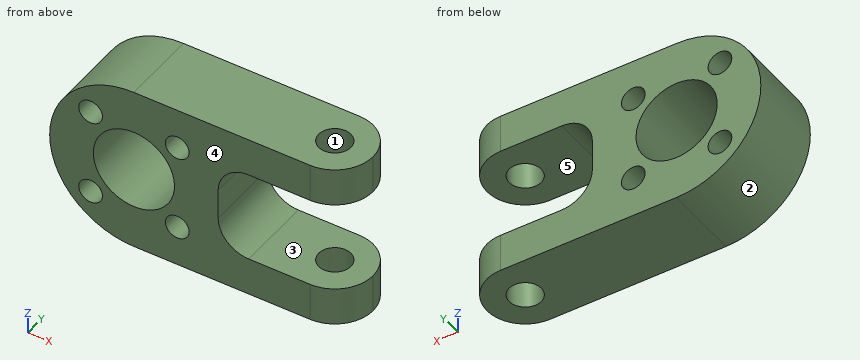
```python
from build123d import *

# Parameters (mm, degrees)
SKETCH2_R           = 5.3
SKETCH2_R_2         = 1.55
BOSS_EXTRUDE2_DEPTH = 10
SKETCH7_R           = 2.1
CUT_EXTRUDE2_DEPTH  = 46.880278988
FILLET1_R           = 4


with BuildPart() as part:
    # Sketch2 → Boss-Extrude2 (new body)
    with BuildSketch(Plane(origin=(0, 0, 0), x_dir=(1, 0, 0), z_dir=(0, 1, 0))):
        with BuildLine():
            Line((-28, -11), (0, -11))
            Line((0, -11), (0, -6))
            Line((0, -6), (-17, -6))
            Line((-17, -6), (-17, 6))
            Line((-17, 6), (0, 6))
            Line((0, 6), (0, 11))
            Line((0, 11), (-28, 11))
            ThreePointArc((-28, 11), (-39, 0), (-28, -11))
        make_face()
        with Locations(Location((-28, 0, 0), (0, 0, 270))):
            Circle(SKETCH2_R, mode=Mode.SUBTRACT)
        with Locations(Location((-33.656854249, 5.656854249, 0), (0, 0, 270))):
            Circle(SKETCH2_R_2, mode=Mode.SUBTRACT)
        with Locations(Location((-33.656854249, -5.656854249, 0), (0, 0, 270))):
            Circle(SKETCH2_R_2, mode=Mode.SUBTRACT)
        with Locations(Location((-22.343145751, 5.656854249, 0), (0, 0, 270))):
            Circle(SKETCH2_R_2, mode=Mode.SUBTRACT)
        with Locations(Location((-22.343145751, -5.656854249, 0), (0, 0, 270))):
            Circle(SKETCH2_R_2, mode=Mode.SUBTRACT)
    extrude(amount=BOSS_EXTRUDE2_DEPTH)

    # Sketch7 → Cut-Extrude2 (cut, through all)
    with BuildSketch(Plane.XY.offset(11)):
        with BuildLine():
            Line((0, 10), (-5, 10))
            ThreePointArc((-5, 10), (-1.464466094, 8.535533906), (0, 5))
            Line((0, 5), (0, 10))
        make_face()
        with BuildLine():
            Line((0, 0), (0, 5))
            ThreePointArc((0, 5), (-1.464466094, 1.464466094), (-5, 0))
            Line((-5, 0), (0, 0))
        make_face()
        with Locations((-5, 5)):
            Circle(SKETCH7_R)
    extrude(amount=-CUT_EXTRUDE2_DEPTH, mode=Mode.SUBTRACT)

    # Fillet1
    fillet1_edges = [part.edges().sort_by_distance(p)[0] for p in [
        (-17, 5, 6),
        (-17, 5, -6),
    ]]
    fillet(fillet1_edges, radius=FILLET1_R)


solid = part.part
```
Geometry check sheet. Reference: the model listing, model coordinates, mm. Face numbers are marked on the shaded views. A direction names the side the tool comes from. Give positions to 0.01 mm unless a question says otherwise; leave off trailing zeros. Order: outer loops, then holes, each group sorted by start corner. A loop starts at its lowest first (then second) coordinate and runs counter-clockwise, first axis right, second up. Notation, with made-up numbers: (54.25, -12.5) - (100.25, -12.5) arc R31 ccw to (100.25, 21.5) - close; hole circle Ø11 at (-26.75, 88). An arc over 180 degrees is marked (long way). Answer in a Markdown table with one row per item. Add a question column.
Q1. Cross-section at C-C, the plane z = -1.5. Enter the section's corners in (x, y), then the cut area to 3 significant figures.
Q2. Material ranges on probe 1 along Z at (x, y) = (-9, 5); probe 2 along Y at (x, z) = (-5, 7.75); probe 3 along Z at (x, y) = (-35, 8), recorded low to high. Write a range as from..to.
Q3. Tool access check on the marked faces 4 and 5. Record the directions out of +Z, -Z, +X, -X, +Y, -Y that give a thin tool (end or side, any length) a straight path to the whole face; none if there is none.
Q4. Cross-section at A-A, the plane y = 9. Enter the section's corners in (x, z).
Q5. Cross-section at D-D, the plane y = 1.75. Enter the section's corners in (x, z).
Q6. Gauge pin test, flat ends, axial feed: pin 1 (8 mm diameter, centred on x = -17, z = -8.5, fed in from -Y); pin 2 (1.9 mm diameter, centred on x = -22.34, z = -5.66, fed in from +Y); pin 3 (4.5 mm diameter, centred on y = 5.5, z = -0.5, fed in from +X). Record the tip position at first contact, or that the pin passes through.
Q7. Cross-section at B-B, the plane x = -14. Enter the section's corners in (y, z).
Q8. Mould release check, pull along Z, two halves, no side actions. Record for the marked faces 1, 2 and 3: pulls with the +Z half, pulls with the -Z half, needs draft (parallel to the pull), parting line crosses it, or undercut.
Check values:
| question | item | result |
|---|---|---|
| 1 | outline | (-38.9, 0) - (-33.08, 0) - (-33.08, 10) - (-38.9, 10) - close; (-22.92, 0) - (-17, 0) - (-17, 10) - (-22.92, 10) - close |
| 1 | area | 117 mm^2 |
| 2 | probe 1 | z = -11..-6, 6..11 |
| 2 | probe 2 | y = 0..2.9, 7.1..10 |
| 2 | probe 3 | z = -8.49..-6.43, -4.88..4.88, 6.43..8.49 |
| 3 | face 4 | +Z, -Z, +X, -X, -Y |
| 3 | face 5 | +X, +Y, -Y |
| 4 | outline | (-28, -11) - (-2, -11) - (-2, -6) - (-13, -6) arc R4 cw to (-17, -2) - (-17, 2) arc R4 cw to (-13, 6) - (-2, 6) - (-2, 11) - (-28, 11) arc R11 ccw to start; hole circle Ø3.1 at (-33.66, -5.66); hole circle Ø3.1 at (-33.66, 5.66); hole circle Ø10.6 at (-28, 0); hole circle Ø3.1 at (-22.34, -5.66); hole circle Ø3.1 at (-22.34, 5.66) |
| 5 | outline | (-28, -11) - (-1.2, -11) - (-1.2, -6) - (-13, -6) arc R4 cw to (-17, -2) - (-17, 2) arc R4 cw to (-13, 6) - (-1.2, 6) - (-1.2, 11) - (-28, 11) arc R11 ccw to start; hole circle Ø3.1 at (-33.66, -5.66); hole circle Ø3.1 at (-33.66, 5.66); hole circle Ø10.6 at (-28, 0); hole circle Ø3.1 at (-22.34, -5.66); hole circle Ø3.1 at (-22.34, 5.66) |
| 6 | pin 1 | stops at y = 0 |
| 6 | pin 2 | passes through |
| 6 | pin 3 | stops at x = -16.93 |
| 7 | outline | (0, -11) - (10, -11) - (10, -5.87) - (0, -5.87) - close; (0, 5.87) - (10, 5.87) - (10, 11) - (0, 11) - close |
| 8 | face 1 | needs draft |
| 8 | face 2 | parting line crosses it |
| 8 | face 3 | undercut |
